```python
from build123d import *

# Parameters (mm, degrees)
SKETCH2_W            = 15.8
SKETCH2_H            = 15.8
BOSS_EXTRUDE2_DEPTH  = 4.2
SKETCH4_W            = 13.4
SKETCH4_H            = 13.4
CUT_EXTRUDE1_DEPTH   = 3
SKETCH6_R            = 2.4
BOSS_EXTRUDE4_DEPTH  = 1.8
LPATTERN1_COUNT      = 2
LPATTERN1_PITCH      = 8
LPATTERN1_COUNT_DIR2 = 2
LPATTERN1_PITCH_DIR2 = 8
SKETCH8_R            = 5.25
CUT_EXTRUDE2_DEPTH   = 0.1
BOSS_EXTRUDE9_DEPTH  = 3
CUT_EXTRUDE3_DEPTH   = 3
CIRPATTERN3_COUNT    = 4
SKETCH19_W           = 1.484523383
SKETCH19_H           = 0.9


with BuildPart() as part:
    # Sketch2 → Boss-Extrude2 (new body)
    with BuildSketch(Plane(origin=(0, 0, 0), x_dir=(1, 0, 0), z_dir=(0, 1, 0))):
        with Locations((7.9, 7.9)):
            Rectangle(SKETCH2_W, SKETCH2_H)
    extrude(amount=-BOSS_EXTRUDE2_DEPTH)

    # Sketch4 → Cut-Extrude1 (cut)
    with BuildSketch(Plane(origin=(0, 0, 0), x_dir=(1, 0, 0), z_dir=(0, 1, 0))):
        with Locations((7.9, 7.9)):
            Rectangle(SKETCH4_W, SKETCH4_H)
    extrude(amount=-CUT_EXTRUDE1_DEPTH, mode=Mode.SUBTRACT)

    # Sketch6 → Boss-Extrude4 (add)
    with BuildSketch(Plane(origin=(0, -4.2, 0), x_dir=(-1, 0, 0), z_dir=(0, -1, 0))):
        with Locations((-11.9, 11.9)):
            Circle(SKETCH6_R)
    boss_extrude4 = extrude(amount=BOSS_EXTRUDE4_DEPTH)

    # LPattern1: Boss-Extrude4 2 × 2
    with Locations(*[(-j * LPATTERN1_PITCH_DIR2, 0, i * LPATTERN1_PITCH) for i in range(LPATTERN1_COUNT) for j in range(LPATTERN1_COUNT_DIR2) if (i, j) != (0, 0)]):
        add(boss_extrude4)

    # Sketch8 → Cut-Extrude2 (cut)
    with BuildSketch(Plane(origin=(0, -3, 0), x_dir=(1, 0, 0), z_dir=(0, 1, 0))):
        with Locations((7.9, 7.9)):
            Circle(SKETCH8_R)
    extrude(amount=-CUT_EXTRUDE2_DEPTH, mode=Mode.SUBTRACT)

    # Sketch11 → Boss-Extrude9 (add)
    with BuildSketch(Plane(origin=(0, -3, 0), x_dir=(1, 0, 0), z_dir=(0, 1, 0))):
        with BuildLine():
            Line((7.899999971, 14.6), (1.2, 14.6))
            Line((1.2, 14.6), (1.2, 7.9))
            ThreePointArc((1.2, 7.9), (3.162384556, 12.637615424), (7.899999971, 14.6))
        make_face()
        with BuildLine():
            Line((14.6, 14.6), (7.899999971, 14.6))
            ThreePointArc((7.899999971, 14.6), (12.637615424, 12.637615444), (14.6, 7.9))
            Line((14.6, 7.9), (14.6, 14.6))
        make_face()
        with BuildLine():
            ThreePointArc((7.900000011, 1.2), (3.16238457, 3.162384562), (1.2, 7.9))
            Line((1.2, 7.9), (1.2, 1.2))
            Line((1.2, 1.2), (7.900000011, 1.2))
        make_face()
        with BuildLine():
            Line((14.6, 1.2), (14.6, 7.9))
            ThreePointArc((14.6, 7.9), (12.637615438, 3.16238457), (7.900000011, 1.2))
            Line((7.900000011, 1.2), (14.6, 1.2))
        make_face()
    extrude(amount=BOSS_EXTRUDE9_DEPTH)

    # Sketch12 → Cut-Extrude3 (cut)
    with BuildSketch(Plane(origin=(0, 0, 0), x_dir=(1, 0, 0), z_dir=(0, 1, 0))):
        Polygon((3.162384566, 12.637615434), (2.455277785, 13.344722215), (1.394617613, 12.284062043), (2.101724394, 11.576955262), align=None)
        with BuildLine():
            ThreePointArc((2.221981276, 11.45669838), (2.658816927, 12.073727351), (3.162384566, 12.637615434))
            Line((3.162384566, 12.637615434), (2.101724394, 11.576955262))
            Line((2.101724394, 11.576955262), (2.221981276, 11.45669838))
        make_face()
        with BuildLine():
            Line((4.223044738, 13.698275606), (3.162384566, 12.637615434))
            ThreePointArc((3.162384566, 12.637615434), (3.726272649, 13.141183073), (4.34330162, 13.578018724))
            Line((4.34330162, 13.578018724), (4.223044738, 13.698275606))
        make_face()
        Polygon((3.515937957, 14.405382387), (2.455277785, 13.344722215), (3.162384566, 12.637615434), (4.223044738, 13.698275606), align=None)
        with BuildLine():
            ThreePointArc((4.34330162, 13.578018724), (3.726272649, 13.141183073), (3.162384566, 12.637615434))
            ThreePointArc((3.162384566, 12.637615434), (2.658816927, 12.073727351), (2.221981276, 11.45669838))
            Line((2.221981276, 11.45669838), (2.423581348, 11.255098309))
            Line((2.423581348, 11.255098309), (4.544901691, 13.376418652))
            Line((4.544901691, 13.376418652), (4.34330162, 13.578018724))
        make_face()
        with BuildLine():
            ThreePointArc((14.6, 7.9), (11.145005458, 13.761735202), (4.34330162, 13.578018724))
            Line((4.34330162, 13.578018724), (4.544901691, 13.376418652))
            Line((4.544901691, 13.376418652), (2.423581348, 11.255098309))
            Line((2.423581348, 11.255098309), (2.221981276, 11.45669838))
            ThreePointArc((2.221981276, 11.45669838), (6.049692654, 1.460561925), (14.6, 7.9))
        make_face()
    cut_extrude3 = extrude(amount=-CUT_EXTRUDE3_DEPTH, mode=Mode.SUBTRACT)

    # CirPattern3: Cut-Extrude3 ×4 about axis
    cirpattern3_axis = Axis((7.9, 0, -7.9), (0, 1, 0))
    for i in range(1, CIRPATTERN3_COUNT):
        add(cut_extrude3.rotate(cirpattern3_axis, i * 360 / CIRPATTERN3_COUNT), mode=Mode.SUBTRACT)

    # Sketch19 → Cut-Revolve1 (revolve, cut)
    with BuildSketch(Plane(origin=(7.9, 0, -7.9), x_dir=(0.707106781, 0, 0.707106781), z_dir=(-0.707106781, 0, 0.707106781))):
        with Locations((-6.957738308, -2.55)):
            Rectangle(SKETCH19_W, SKETCH19_H)
    revolve(axis=Axis((7.9, 0, -7.9), (0, -1, 0)), mode=Mode.SUBTRACT)


solid = part.part
```
Check sheet for the modelled part. Datum: model origin and axes. Units: mm. A direction names the side the tool comes from. Coordinates: 2 decimals unless noted, no trailing zeros. Write each loop counter-clockwise with the first axis right and the second up, starting at its lowest first coordinate (ties: lowest second). Pieces come first, ordered by that corner, then holes. Notation, with made-up numbers: (-39, 79.5) -> (18, 79.5) arc R22 cw to (18, 118.5) -> close; hole circle Ø7 at (62, 13). An arc over 180 degrees is marked (long way). Use a Markdown table: item, result.
1. Sectioned sample at B-B (x = 3.9). Enter the section's corners in (y, z).
Reported:
| item | result |
|---|---|
| outline | (-6, -14.3) -> (-4.2, -14.3) -> (-4.2, -15.8) -> (0, -15.8) -> (0, -14.02) -> (-2.1, -14.02) -> (-2.1, -14.48) -> (-3, -14.48) -> (-3, -11.3) -> (-3.1, -11.3) -> (-3.1, -4.5) -> (-3, -4.5) -> (-3, -1.32) -> (-2.1, -1.32) -> (-2.1, -1.78) -> (0, -1.78) -> (0, 0) -> (-4.2, 0) -> (-4.2, -1.5) -> (-6, -1.5) -> (-6, -6.3) -> (-4.2, -6.3) -> (-4.2, -9.5) -> (-6, -9.5) -> close |
2. Sectioned sample at C-C (z = -1). Enter the section's corners in (x, y), plus the area to 3 significant figures.
Reported:
| item | result |
|---|---|
| outline | (0, -4.2) -> (15.8, -4.2) -> (15.8, 0) -> (0, 0) -> close; hole (4.48, -3) -> (11.32, -3) -> (11.32, -2.1) -> (4.48, -2.1) -> close |
| area | 60.2 mm2 |
3. Sectioned sample at D-D (y = -4.55). Enter the section's corners in (x, z), plus the area to 3 significant figures.
Reported:
| item | result |
|---|---|
| outline | circle Ø4.8 at (3.9, -11.9); circle Ø4.8 at (3.9, -3.9); circle Ø4.8 at (11.9, -11.9); circle Ø4.8 at (11.9, -3.9) |
| area | 72.4 mm2 |
4. Sectioned sample at A-A (y = -0.4). Enter the section's corners in (x, z).
Reported:
| item | result |
|---|---|
| outline | (0, -15.8) -> (15.8, -15.8) -> (15.8, 0) -> (0, 0) -> close; hole (1.39, -12.28) -> (3.52, -14.41) -> (4.34, -13.58) arc R6.7 ccw to (11.46, -13.58) -> (12.28, -14.41) -> (14.41, -12.28) -> (13.58, -11.46) arc R6.7 ccw to (13.58, -4.34) -> (14.41, -3.52) -> (12.28, -1.39) -> (11.46, -2.22) arc R6.7 ccw to (4.34, -2.22) -> (3.52, -1.39) -> (1.39, -3.52) -> (2.22, -4.34) arc R6.7 ccw to (2.22, -11.46) -> close |
5. Scan lines: line 1 along Z through (x, y) = (7.9, -3.05); line 2 along Y through (x, z) = (6.25, -14.5); line 3 along Z through (x, y) = (13.75, -1.9). Record each from-to range of solid material in increasing order.
Reported:
| item | result |
|---|---|
| line 1 | z = -15.8 to -13.15, -2.65 to 0 |
| line 2 | y = -4.2 to -3, -2.1 to 0 |
| line 3 | z = -15.8 to -12.94, -11.63 to -11.17, -4.63 to -4.17, -2.86 to 0 |
6. Tool access check on faces 1 (the flat face through (3.935, -1.146, -13.986)), 2 (the cylindrical face through (0.2, -2.5, -7.8)), 3 (the cylindrical face through (2.79, -5.09, -1.77)). Record the directions out of +Z, -Z, +X, -X, +Y, -Y that give a thin tool (end or side, any length) a straight path to the whole face; none if there is none.
Reported:
| item | result |
|---|---|
| face 1 | +Y |
| face 2 | none |
| face 3 | -Y |
7. Go/stop test with flat-tipped pins: pin 1 Ø3 at (x, z) = (10.5, -6) entering from +Y; pin 2 Ø1.6 at (x, z) = (15, -7.5) entering from -Y. Record where each tip stops, or that it passes through.
Reported:
| item | result |
|---|---|
| pin 1 | stops at y = -3.1 |
| pin 2 | stops at y = -4.2 |
8. Release check for a two-part mould opening along Z. For faces 4 (the flat face through (8, -2, -15.8)), 5 (the flat face through (13, -3, -6)), 6 (the flat face through (4, -6, -12)), 7 (the flat face through (8, -2, 0)) record: pulls with the +Z half, pulls with the -Z half, needs draft (parallel to the pull), parting line crosses it, or undercut.
Reported:
| item | result |
|---|---|
| face 4 | pulls with the -Z half |
| face 5 | undercut |
| face 6 | needs draft |
| face 7 | pulls with the +Z half |
